Could you check a few things on this drawing? It's one solid part, dimensions in mm from its lowest x, y, z. A direction names the side the tool comes from. Give positions to 0.01 mm unless a question says otherwise; leave off trailing zeros. Loops run counter-clockwise (first coordinate to the right, second up) from the corner with the lowest first, then second, coordinate; pieces in that order, holes last.
Q1. Suppose I cut it at A-A (x = 13). List the corners of the cut face in (y, z) for me, and give its area (3 significant figures).
Q2. I'm going to push flat-ended pins straight in: P1, Ø12, axis at x = 5.5, z = 19.5, coming from the -Y side; P2, Ø12, axis at x = 26.5, z = 8.5, coming from the -Y side; P3, Ø2, axis at x = 25, y = 31, coming from the +Z side. Where does each tip first touch, or does it pass through?
Q3. Suppose I cut it at C-C (z = 26). List the corners of the cut face in (x, y) for me, and give its area (3 significant figures).
Q4. Suppose I cut it at D-D (z = 8.5). List the corners of the cut face in (x, y) for me, and give its area (3 significant figures).
Q5. For the marked faces 1, 2 and 3, which set-ups out of +Z, -Z, +X, -X, +Y, -Y let a thin tool reach every point of the face, with its end or its side?
Q6. I need wall thicknesses on probe 1 along Y at (x, z) = (8, 21.5); probe 2 along X at (y, z) = (27, 22.5); probe 3 along Z at (x, y) = (29.5, 22.5). Which ranges of each line are inside material? Lowest first, please.
Q7. Suppose I cut it at B-B (y = 29). List the corners of the cut face in (x, z) for me.
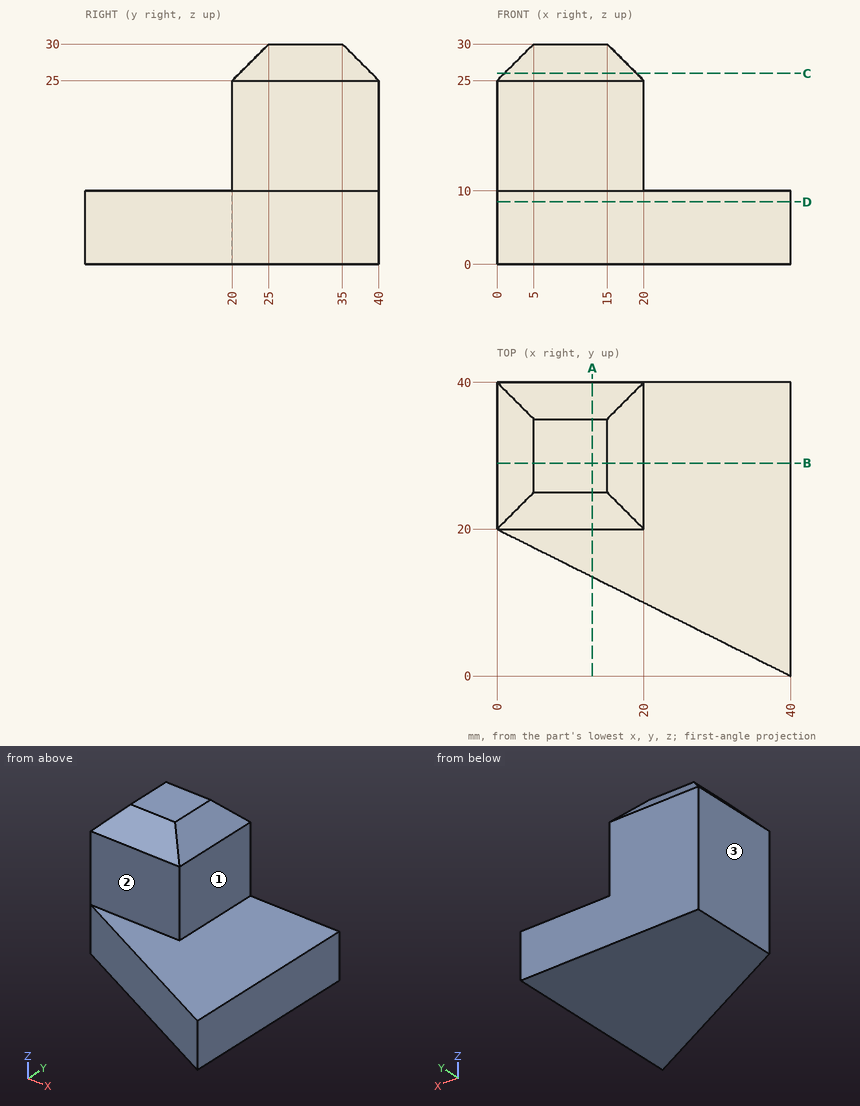
Solutions:
1. outline: (13.5, 0) - (40, 0) - (40, 25) - (35, 30) - (25, 30) - (20, 25) - (20, 10) - (13.5, 10) - close
1. area: 640 mm2
2. P1: stops at y = 20
2. P2: stops at y = 3.75
2. P3: stops at z = 10
3. outline: (1, 21) - (19, 21) - (19, 39) - (1, 39) - close
3. area: 324 mm2
4. outline: (0, 20) - (40, 0) - (40, 40) - (0, 40) - close
4. area: 1,200 mm2
5. face 1: +Z, +X, +Y, -Y
5. face 2: +Z, +X, -X, -Y
5. face 3: +Z, -Z, -X, +Y, -Y
6. probe 1: y = 20 to 40
6. probe 2: x = 0 to 20
6. probe 3: z = 0 to 10
7. outline: (0, 0) - (40, 0) - (40, 10) - (20, 10) - (20, 25) - (15, 30) - (5, 30) - (0, 25) - close
